```python
from build123d import *

# Parameters (mm, degrees)
F0_W     = 78.5
F0_H     = 75
F1_DEPTH = 4.8
F2_R     = 5.2
F2_R_2   = 5.59
F2_R_3   = 3.3
F2_W     = 2.9
F2_H     = 2.9
F3_DEPTH = 4.801
F4_R     = 10
F5_DEPTH = 2.5
F6_R     = 2


with BuildPart() as f1:
    # F0 (on Front) → F1 (new body)
    with BuildSketch(Plane.XZ):
        Rectangle(F0_W, F0_H)
    extrude(amount=F1_DEPTH)

    # F2 (on face) → F3 (cut, through all)
    with BuildSketch(Plane.XZ.offset(4.8)):
        with Locations((-27.25, 0)):
            Circle(F2_R)
        with Locations((-27.25, -19.91)):
            Circle(F2_R_2)
        with Locations((-2.25, -19.91)):
            Circle(F2_R_2)
        with Locations((-2.25, 0)):
            Circle(F2_R)
        with Locations((0, 22.2)):
            Circle(F2_R_3)
        with Locations((-20, 22.2)):
            Circle(F2_R_3)
        with Locations((20, 22.2)):
            Circle(F2_R_3)
        with Locations((17.9, 3.948761)):
            Rectangle(F2_W, F2_H)
        with Locations((27.8, 3.948761)):
            Rectangle(F2_W, F2_H)
        with Locations((17.9, -5.951239)):
            Rectangle(F2_W, F2_H)
        with Locations((27.8, -5.951239)):
            Rectangle(F2_W, F2_H)
        with Locations((17.9, -19.91)):
            Rectangle(F2_W, F2_H)
        with Locations((27.8, -19.91)):
            Rectangle(F2_W, F2_H)
    extrude(amount=-F3_DEPTH, mode=Mode.SUBTRACT)

    # F4 (on face) → F5 (cut)
    with BuildSketch(Plane(origin=(0, 0, 0), x_dir=(-1, 0, 0), z_dir=(0, 1, 0))):
        with Locations((2.25, 0)):
            Circle(F4_R)
        with Locations((27.25, 0)):
            Circle(F4_R)
    extrude(amount=-F5_DEPTH, mode=Mode.SUBTRACT)

    # F6
    f6_edges = [f1.edges().sort_by_distance(p)[0] for p in [
        (7.75, -2.5, 0),
        (-17.25, -2.5, 0),
    ]]
    fillet(f6_edges, radius=F6_R)


solid = f1.part
```
Model file for the job. Use its own axes, mm. A direction names the side the tool comes from. Coordinates: 2 decimals unless noted, no trailing zeros. Order: outer loops, then holes, each group sorted by start corner. A loop starts at its lowest first (then second) coordinate and runs counter-clockwise, first axis right, second up. Notation, with made-up numbers: (58, 81.25) -> (81, 81.25) arc R15 cw to (81, 96.25) -> close; hole circle Ø11 at (17.25, -4). An arc over 180 degrees is marked (long way). Return JSON: item names as keys, results as strings.
Item 1: 3-axis set-ups, long thin cutter, end or side, ignore diameter. For faces 3 (the face through (16.45, -2, -6)), 4 (the face through (-11.79, -0.25, 3)): which of +Z, -Z, +X, -X, +Y, -Y reach the whole face in a straight line?
Model answer:
{"face 3": "+Y, -Y", "face 4": "+Y"}
Item 2: Slice it at C-C (z = 0). Write the cut outline in (x, y), then the cut area to 3 significant figures.
Model answer:
{"outline": "(-39.25, -4.8) -> (-32.45, -4.8) -> (-32.45, -2.5) -> (-35.25, -2.5) arc R2 cw to (-37.25, -0.5) -> (-37.25, 0) -> (-39.25, 0) -> close; (-22.05, -4.8) -> (-7.45, -4.8) -> (-7.45, -2.5) -> (-10.25, -2.5) arc R2 cw to (-12.25, -0.5) -> (-12.25, 0) -> (-17.25, 0) -> (-17.25, -0.5) arc R2 cw to (-19.25, -2.5) -> (-22.05, -2.5) -> close; (2.95, -4.8) -> (39.25, -4.8) -> (39.25, 0) -> (7.75, 0) -> (7.75, -0.5) arc R2 cw to (5.75, -2.5) -> (2.95, -2.5) -> close", "area": "232 mm²"}
Item 3: Slice it at B-B (x = -27.25). Write the cut outline in (y, z), then the cut area to 3 significant figures.
Model answer:
{"outline": "(-4.8, -37.5) -> (0, -37.5) -> (0, -25.5) -> (-4.8, -25.5) -> close; (-4.8, -14.32) -> (0, -14.32) -> (0, -10) -> (-0.5, -10) arc R2 cw to (-2.5, -8) -> (-2.5, -5.2) -> (-4.8, -5.2) -> close; (-4.8, 5.2) -> (-2.5, 5.2) -> (-2.5, 8) arc R2 cw to (-0.5, 10) -> (0, 10) -> (0, 37.5) -> (-4.8, 37.5) -> close", "area": "234 mm²"}
Item 4: Wall check: line 1 along Z through (x, y) = (-27.25, -3.95); line 2 along X through (y, z) = (-4.6, -4); line 3 along X through (y, z) = (-1.55, 8.5). Give the ranges that are in metal, low to high. Write a range as from..to.
Model answer:
{"line 1": "z = -37.5..-25.5, -14.32..-5.2, 5.2..37.5", "line 2": "x = -39.25..-30.57, -23.93..-5.57, 1.07..39.25", "line 3": "x = -39.25..-31.93, -22.57..-6.93, 2.43..39.25"}
Item 5: Pin check, flat tips, straight feed: P1, Ø3, axis at x = -11, z = -17, coming from the +Y side; P2, Ø16.5, axis at x = -2.25, z = 0, coming from the +Y side. Stop position of each tip, or through.
Model answer:
{"P1": "stops at y = 0", "P2": "stops at y = -2.48"}
Item 6: Mould opens along Z. For faces 1 (the face through (-1, -2, -37.5)), 2 (the face through (-22.086, -2.434, -22.051)) say: pulls with the +Z half, pulls with the -Z half, needs draft (parallel to the pull), parting line crosses it, or undercut.
Model answer:
{"face 1": "pulls with the -Z half", "face 2": "undercut"}
Item 7: Slice it at A-A (z = -19.91). Write the cut outline in (x, y).
Model answer:
{"outline": "(-39.25, -4.8) -> (-32.84, -4.8) -> (-32.84, 0) -> (-39.25, 0) -> close; (-21.66, -4.8) -> (-7.84, -4.8) -> (-7.84, 0) -> (-21.66, 0) -> close; (3.34, -4.8) -> (16.45, -4.8) -> (16.45, 0) -> (3.34, 0) -> close; (19.35, -4.8) -> (26.35, -4.8) -> (26.35, 0) -> (19.35, 0) -> close; (29.25, -4.8) -> (39.25, -4.8) -> (39.25, 0) -> (29.25, 0) -> close"}
Item 8: Slice it at D-D (y = -3.4). Count the separate pieces of the cut face and the enclosed holes in it, then the cut area to 3 significant figures.
Model answer:
{"separate pieces": "1", "enclosed holes": "13", "area": "5,370 mm²"}
